Autodesk Inventor part; units mm, degrees
ref_plane "YZ Plane" through (0, 0, 0) normal (1, 0, 0) x (0, 1, 0)
ref_plane "XZ Plane" through (0, 0, 0) normal (0, 1, 0) x (-1, 0, 0)
ref_plane "XY Plane" through (0, 0, 0) normal (0, 0, 1) x (1, 0, 0)
sketch "Boceto1" plane through (0, 0, 0) normal (0, 0, 1) x (1, 0, 0)
  line L0 (0, 5) -> (0, 165)
  line L1 (5, 170) -> (30, 170)
  line L2 (35, 165) -> (35, 5)
  line L3 (30, 0) -> (5, 0)
  arc A0 (35, 165) -> (30, 170) centre (30, 165) ccw
  arc A1 (5, 170) -> (0, 165) centre (5, 165) ccw
  arc A2 (0, 5) -> (5, 0) centre (5, 5) ccw
  arc A3 (30, 0) -> (35, 5) centre (30, 5) ccw
  circle A4 centre (17.5, 140) radius 4.5
  circle A5 centre (17.5, 120) radius 2.5
  circle A6 centre (17.5, 100) radius 2.5
  circle A7 centre (17.5, 80) radius 2.5
  circle A8 centre (17.5, 20) radius 2.5
  circle A9 centre (6, 133) radius 1.25
  circle A10 centre (6, 146.5) radius 1.25
  circle A11 centre (29, 146.5) radius 1.25
  circle A12 centre (29, 133) radius 1.25
  point P0 (0, 0)
extrude "Extrusión1" add sketch "Boceto1" along normal blind 3
properties part number "2"
CAD build for the part. Positions are in the model's coordinates, mm. Coordinates: 2 decimals unless noted, no trailing zeros. Write each loop counter-clockwise with the first axis right and the second up, starting at its lowest first coordinate (ties: lowest second). Pieces come first, ordered by that corner, then holes.
(1) Cut at A-A, the plane y = 140. List the corners of the cut face in (x, z).
(2) Drill centre lines: probe 1 along Y at (x, z) = (6, 1.5); probe 2 along Y at (x, z) = (17.5, 1.7); probe 3 along X at (y, z) = (146.5, 1.85). Where is each one in solid material? Low to high.
(3) Cut at B-B, the plane x = 17.5. List the corners of the cut face in (y, z).
(4) Cut at D-D, the plane y = 20. List the corners of the cut face in (x, z), and give its area (3 significant figures).
(5) Cut at C-C, the plane z = 1.6. Count the separate pieces of the cut face and the enclosed holes in it, and give its area (3 significant figures).
(6) Flat gauge pin, fed straight in: pin 1 (6 mm diameter, centred on x = 17.5, y = 120, fed in from -Z). Where does the tip first touch, or does it go through?
(7) Two-plate mould, pull along Y, no slides. Class faces 1 (the face through (17, 86, 3)), 2 (the face through (17.17, 97.52, 1.48)), 3 (the face through (33, 169, 1)), 4 (the face through (17.17, 117.52, 1.48)): +Y half, -Y half, draft (parallel to the pull), parting line (faces both ways), or undercut.
Geometry says:
1. outline: (0, 0) - (13, 0) - (13, 3) - (0, 3) - close; (22, 0) - (35, 0) - (35, 3) - (22, 3) - close
2. probe 1: y = 0 to 131.75, 134.25 to 145.25, 147.75 to 170
2. probe 2: y = 0 to 17.5, 22.5 to 77.5, 82.5 to 97.5, 102.5 to 117.5, 122.5 to 135.5, 144.5 to 170
2. probe 3: x = 0 to 4.75, 7.25 to 27.75, 30.25 to 35
3. outline: (0, 0) - (17.5, 0) - (17.5, 3) - (0, 3) - close; (22.5, 0) - (77.5, 0) - (77.5, 3) - (22.5, 3) - close; (82.5, 0) - (97.5, 0) - (97.5, 3) - (82.5, 3) - close; (102.5, 0) - (117.5, 0) - (117.5, 3) - (102.5, 3) - close; (122.5, 0) - (135.5, 0) - (135.5, 3) - (122.5, 3) - close; (144.5, 0) - (170, 0) - (170, 3) - (144.5, 3) - close
4. outline: (0, 0) - (15, 0) - (15, 3) - (0, 3) - close; (20, 0) - (35, 0) - (35, 3) - (20, 3) - close
4. area: 90.0 mm2
5. separate pieces: 1
5. enclosed holes: 9
5. area: 5,770 mm2
6. pin 1: stops at z = 0
7. face 1: draft
7. face 2: undercut
7. face 3: +Y half
7. face 4: undercut
